Geometry: final body of the model. Coordinates: model frame, mm. A direction names the side the tool comes from. Round coordinates to 2 decimals unless told otherwise and drop trailing zeros. Order: outer loops, then holes, each group sorted by start corner. A loop starts at its lowest first (then second) coordinate and runs counter-clockwise, first axis right, second up. Notation, with made-up numbers: M 11.25,3 L 49.25,3 A25 cw 49.25,25 Z; hole C 89.5,8.5 d4. An arc over 180 degrees is marked long. Put each result on its own line as item: value. Start each with the question number.
1) Section C-C, the plane y = 387.5. Count the separate pieces of the cut face and the enclosed holes in it, then the cut area to 3 significant figures.
2) Section A-A, the plane z = 29. Return loops of the section in (x, y).
3) Section D-D, the plane z = -75.5. Return loops of the section in (x, y), then the cut area to 3 significant figures.
4) Draft query along Y for faces 5 (the flat face through (441.5, 6, 20)), 6 (the cylindrical face through (76.09, -342.653, -80.28)), 7 (the cylindrical face through (-381.53, 120.15, -55.63)). Return one class per face: pulls with the +Y half, pulls with the -Y half, needs draft (parallel to the pull), parting line crosses it, or undercut.
5) Section B-B, the plane x = -421.5. Return loops of the section in (y, z).
6) First-contact query: P1, Ø1, axis at y = 114.5, z = 42.5, coming from the +X side; P2, Ø5, axis at x = -90, z = 74.5, coming from the +Y side; P3, Ø11, axis at x = 14.5, y = -413, coming from the +Z side; P4, Ø12, axis at x = 421.5, y = 387.5, coming from the +Z side. Flat tips, straight axial feed; report the tip coordinate or a pass-through.
7) Material intervals for probe 1 along Y at (x, z) = (-421, -7); probe 2 along Y at (x, z) = (0, 11); probe 3 along X at (y, z) = (-156, 35), sorted ascending. Write a range as [from, to].
8) Access query for faces 1 (the cylindrical face through (-380.575, 119.849, -79.72)), 2 (the flat face through (-2, 404, 0)), 3 (the cylindrical face through (-411.96, 390.5, -4.93)), 4 (the flat face through (-441.5, 6, 20)). Directions: +Z, -Z, +X, -X, +Y, -Y. A direction counts if a zero-diameter tool reaches every point of the face in a straight line with its end or side. Return the directions, or none.
from build123d import *

# Parameters (mm, degrees)
F2_W     = 903
F2_H     = 835
F2_R     = 10
F2_R_2   = 400
F3_DEPTH = 10
F4_W     = 793
F4_H     = 10
F4_W_2   = 10
F4_H_2   = 835
F5_DEPTH = 50


with BuildPart() as f1:
    # F0 (on Front) → F1 (revolve)
    with BuildSketch(Plane.XZ):
        Polygon((-351, -100), (-350, -100), (-350, 55), (-351, 55), (-351, 95), (-399, 95), (-399, 55), (-400, 55), (-400, -100), (-399, -100), (-399, -60), (-351, -60), align=None)
    revolve(axis=Axis((0, 0, -77.049306), (0, 0, -1)))

    # F2 (on Top) → F3 (join)
    with BuildSketch(Plane.XY):
        Rectangle(F2_W, F2_H)
        with Locations((-421.5, -387.5)):
            Circle(F2_R, mode=Mode.SUBTRACT)
        with Locations((421.5, -387.5)):
            Circle(F2_R, mode=Mode.SUBTRACT)
        with Locations((-421.5, 387.5)):
            Circle(F2_R, mode=Mode.SUBTRACT)
        Circle(F2_R_2, mode=Mode.SUBTRACT)
        with Locations((421.5, 387.5)):
            Circle(F2_R, mode=Mode.SUBTRACT)
    extrude(amount=-F3_DEPTH)

    # F4 (on face) → F5 (join)
    with BuildSketch(Plane(origin=(0, 0, -10), x_dir=(1, 0, 0), z_dir=(0, 0, -1))):
        with Locations((0, 412.5)):
            Rectangle(F4_W, F4_H)
        with Locations((-446.5, 0)):
            Rectangle(F4_W_2, F4_H_2)
        with Locations((0, -412.5)):
            Rectangle(F4_W, F4_H)
        with Locations((446.5, 0)):
            Rectangle(F4_W_2, F4_H_2)
    extrude(amount=-F5_DEPTH)


solid = f1.part
Result sheet:
1. separate pieces: 3
1. enclosed holes: 0
1. area: 38,200 mm2
2. outline: M -451.5,-417.5 L -441.5,-417.5 L -441.5,417.5 L -451.5,417.5 Z; C 0,0 d800; M -396.5,-417.5 L 396.5,-417.5 L 396.5,-407.5 L -396.5,-407.5 Z; M -396.5,407.5 L 396.5,407.5 L 396.5,417.5 L -396.5,417.5 Z; M 441.5,-417.5 L 451.5,-417.5 L 451.5,417.5 L 441.5,417.5 Z; hole C 0,0 d700
3. outline: C 0,0 d800; C 0,0 d702; hole C 0,0 d798; hole C 0,0 d700
3. area: 4,710 mm2
4. face 5: needs draft
4. face 6: undercut
4. face 7: parting line crosses it
5. outline: M -417.5,-10 L -397.5,-10 L -397.5,0 L -417.5,0 Z; M -377.5,-10 L 377.5,-10 L 377.5,0 L -377.5,0 Z; M 397.5,-10 L 417.5,-10 L 417.5,0 L 397.5,0 Z
6. P1: stops at x = 383.41
6. P2: stops at y = 389.29
6. P3: stops at z = 40
6. P4: passes through
7. probe 1: y = [-417.5, -397.49], [-377.51, 377.51], [397.49, 417.5]
7. probe 2: y = [-417.5, -407.5], [-400, -350], [350, 400], [407.5, 417.5]
7. probe 3: x = [-451.5, -441.5], [-368.33, -313.31], [313.31, 368.33], [441.5, 451.5]
8. face 1: -Z
8. face 2: +Z
8. face 3: +Z, -Z
8. face 4: +Z, +Y, -Y
